Input: part model. Units: mm. Frame: model coordinates. Face numbers are marked on the shaded views. A direction names the side the tool comes from. Coordinates: 2 decimals unless noted, no trailing zeros. Write each loop counter-clockwise with the first axis right and the second up, starting at its lowest first coordinate (ties: lowest second). Pieces come first, ordered by that corner, then holes.
1) Section query A-A (y = 6.5). Output: boundary loops of the cut face in (x, z), then the cut area to 3 significant figures.
2) Pin query (flat end, axial travel): pin 1 Ø9 at (x, z) = (-4, -7) entering from -Y; pin 2 Ø1 at (x, z) = (-5.5, 7.5) entering from -Y; pin 3 Ø3 at (x, y) = (8, 6) entering from -Z; pin 4 Ø3.5 at (y, z) = (8, -21.5) entering from +X. Return the tip coordinate at first contact, or that it passes through.
3) Draft query along X for the marked faces 4, 5 and 6. Return one class per face: pulls with the +X half, pulls with the -X half, needs draft (parallel to the pull), parting line crosses it, or undercut.
4) Section query B-B (z = 21). Output: boundary loops of the cut face in (x, y), then the cut area to 3 significant figures.
5) Section query C-C (y = 11.75). Output: boundary loops of the cut face in (x, z), then the cut area to 3 significant figures.
6) Line query: L1, parallel to Y at x = -13, z = -21; L2, parallel to Z at x = 0, y = 4; L3, parallel to Z at x = -13.5, y = 6.75. Output: solid intervals per line, ascending.
7) Set-up query: the marked faces 1, 2 and 3. Return all of +Z, -Z, +X, -X, +Y, -Y with unobstructed straight access to the full face (end or side cutting, diameter ignored); none if empty.
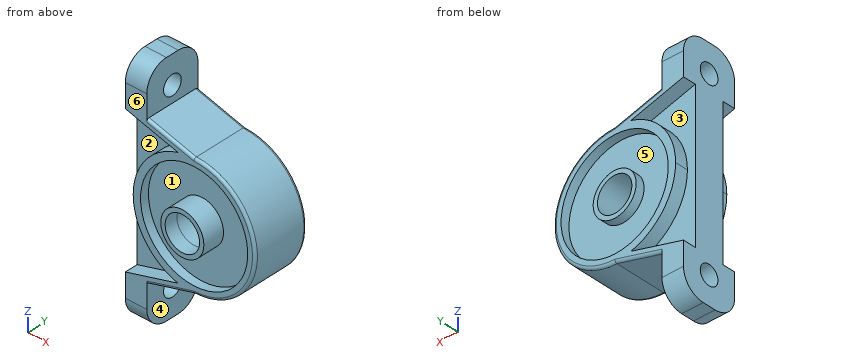
from build123d import *

# Parameters (mm, degrees)
SKETCH_1_R          = 14.162262157
SKETCH_1_R_2        = 12.458976409
SKETCH_1_R_3        = 5
SKETCH_1_R_4        = 4
EXTRUDE_1_DEPTH     = 13
EXTRUDE_START       = 2
SKETCH_1_3_R        = 12.458976409
SKETCH_1_3_R_2      = 5
EXTRUDE_2_DEPTH     = 9
SKETCH_2_R          = 2.25
CUT_EXTRUDE_1_DEPTH = 9
FILLET_1_R          = 5
EXTRUDE_START_2     = 3
SKETCH_3_R          = 5
SKETCH_3_R_2        = 4
EXTRUDE_3_DEPTH     = 3
CUT_EXTRUDE_2_DEPTH = 3
FILLET_2_R          = 0.6


with BuildPart() as part:
    # Sketch 1 → Extrude 1 (new body)
    # profile 1 of 3: a face of its own
    with BuildSketch(Plane(origin=(0, 0, 0), x_dir=(1, 0, 0), z_dir=(0, 1, 0))):
        with BuildLine():
            Line((-11, 27.5), (-16, 27.5))
            Line((-16, 27.5), (-16, -27.5))
            Line((-16, -27.5), (-11, -27.5))
            Line((-11, -27.5), (-11, -17.206839795))
            Line((-11, -17.206839795), (0, -14.162262157))
            ThreePointArc((0, -14.162262157), (-14.162262157, 0), (0, 14.162262157))
            Line((0, 14.162262157), (-11, 17.206839795))
            Line((-11, 17.206839795), (-11, 27.5))
        make_face()
    # profile 2 of 3: a face of its own
    with BuildSketch(Plane(origin=(0, 0, 0), x_dir=(1, 0, 0), z_dir=(0, 1, 0))):
        Circle(SKETCH_1_R)
        with Locations(Location((0, 0, 0), (0, 0, 90))):
            Circle(SKETCH_1_R_2, mode=Mode.SUBTRACT)
    # profile 3 of 3: a face of its own
    with BuildSketch(Plane(origin=(0, 0, 0), x_dir=(1, 0, 0), z_dir=(0, 1, 0))):
        with Locations(Location((0, 0, 0), (0, 0, 90))):
            Circle(SKETCH_1_R_3)
        with Locations(Location((0, 0, 0), (0, 0, 90))):
            Circle(SKETCH_1_R_4, mode=Mode.SUBTRACT)
    extrude(amount=EXTRUDE_1_DEPTH)

    # Sketch 1_3 → Extrude 2 (add)
    with BuildSketch(Plane(origin=(0, 0, 0), x_dir=(1, 0, 0), z_dir=(0, 1, 0)).offset(EXTRUDE_START)):
        with Locations(Location((0, 0, 0), (0, 0, 90))):
            Circle(SKETCH_1_3_R)
        with Locations(Location((0, 0, 0), (0, 0, 90))):
            Circle(SKETCH_1_3_R_2, mode=Mode.SUBTRACT)
    extrude(amount=EXTRUDE_2_DEPTH)

    # Sketch 2 → Cut-Extrude 1 (cut)
    with BuildSketch(Plane(origin=(-11, 0, 0), x_dir=(0, 0, -1), z_dir=(1, 0, 0))):
        with Locations((21, 6.5)):
            Circle(SKETCH_2_R)
        with Locations((-21, 6.5)):
            Circle(SKETCH_2_R)
    extrude(amount=-CUT_EXTRUDE_1_DEPTH, mode=Mode.SUBTRACT)

    # Fillet 1
    fillet_1_edges = [part.edges().sort_by_distance(p)[0] for p in [
        (-13.5, 0, 27.5),
        (-13.5, 0, -27.5),
        (-13.5, 13, -27.5),
        (-13.5, 13, 27.5),
    ]]
    fillet(fillet_1_edges, radius=FILLET_1_R)

    # Sketch 3 → Extrude 3 (add)
    with BuildSketch(Plane.XZ.offset(EXTRUDE_START_2)):
        with Locations(Location((0, 0, 0), (0, 0, 270))):
            Circle(SKETCH_3_R)
        with Locations(Location((0, 0, 0), (0, 0, 270))):
            Circle(SKETCH_3_R_2, mode=Mode.SUBTRACT)
    extrude(amount=-EXTRUDE_3_DEPTH)

    # Sketch 4 → Cut-Extrude 2 (cut)
    with BuildSketch(Plane.XZ):
        with BuildLine():
            Line((-16, 0), (-16, -17.034343572))
            Line((-16, -17.034343572), (-3.773486703, -13.650291847))
            ThreePointArc((-3.773486703, -13.650291847), (-11.26966675, -8.576962209), (-14.162262157, 0))
            Line((-14.162262157, 0), (-16, 0))
        make_face()
        with BuildLine():
            Line((-16, 17.034343572), (-16, 0))
            Line((-16, 0), (-14.162262157, 0))
            ThreePointArc((-14.162262157, 0), (-11.26966675, 8.576962209), (-3.773486703, 13.650291847))
            Line((-3.773486703, 13.650291847), (-16, 17.034343572))
        make_face()
    cut_extrude_2 = extrude(amount=-CUT_EXTRUDE_2_DEPTH, mode=Mode.SUBTRACT)

    # Mirror 1: Cut-Extrude 2 across plane
    add(cut_extrude_2.mirror(Plane.ZX.offset(6.5)), mode=Mode.SUBTRACT)

    # Fillet 2
    fillet_2_edges = [part.edges().sort_by_distance(p)[0] for p in [
        (-5.5, 0, -15.684550976),
        (-5.5, 13, -15.684550976),
        (14.162262157, 0, 0),
        (-5.5, 0, 15.684550976),
        (-5.5, 13, 15.684550976),
        (14.162262157, 13, 0),
    ]]
    fillet(fillet_2_edges, radius=FILLET_2_R)


solid = part.part
Answer:
1. outline: (-16, -27.5) - (-11, -27.5) - (-11, -23.25) - (-16, -23.25) - close; (-16, -18.75) - (-11, -18.75) - (-11, -17.21) - (0, -14.16) arc R14.16 ccw to (0, 14.16) - (-11, 17.21) - (-11, 18.75) - (-16, 18.75) - close; (-16, 23.25) - (-11, 23.25) - (-11, 27.5) - (-16, 27.5) - close; hole circle Ø8 at (0, 0)
1. area: 840 mm2
2. pin 1: stops at y = -3
2. pin 2: stops at y = 2
2. pin 3: stops at z = -12.58
2. pin 4: stops at x = -11
3. face 4: pulls with the +X half
3. face 5: undercut
3. face 6: needs draft
4. outline: (-16, 0) - (-11, 0) - (-11, 4.25) - (-16, 4.25) - close; (-16, 8.75) - (-11, 8.75) - (-11, 13) - (-16, 13) - close
4. area: 42.5 mm2
5. outline: (-16, -25.81) - (-11, -25.81) - (-11, -17.21) - (0, -14.16) arc R14.16 ccw to (0, 14.16) - (-11, 17.21) - (-11, 25.81) - (-16, 25.81) - (-16, 17.03) - (-3.77, 13.65) arc R14.16 ccw to (-3.77, -13.65) - (-16, -17.03) - close; circle Ø10 at (0, 0); hole circle Ø24.92 at (0, 0); hole circle Ø8 at (0, 0)
5. area: 293 mm2
6. L1: y = 0 to 4.25, 8.75 to 13
6. L2: z = -14.16 to -4, 4 to 14.16
6. L3: z = -27.5 to -23.24, -18.76 to 18.76, 23.24 to 27.5
7. face 1: -Y
7. face 2: -X, -Y
7. face 3: -X, +Y
